For this review, take the finished solid that the model builds, in its own axes (mm). Face numbers are marked on the shaded views. Round coordinates to 2 decimals unless told otherwise and drop trailing zeros. Write each loop counter-clockwise with the first axis right and the second up, starting at its lowest first coordinate (ties: lowest second). Pieces come first, ordered by that corner, then holes. Notation, with made-up numbers: M 45,-28.75 L 58,-28.75 A16 cw 58,-7.75 Z; hole C 39.25,-38.5 d4. An arc over 180 degrees is marked long. Answer in a Markdown table with one row per item.
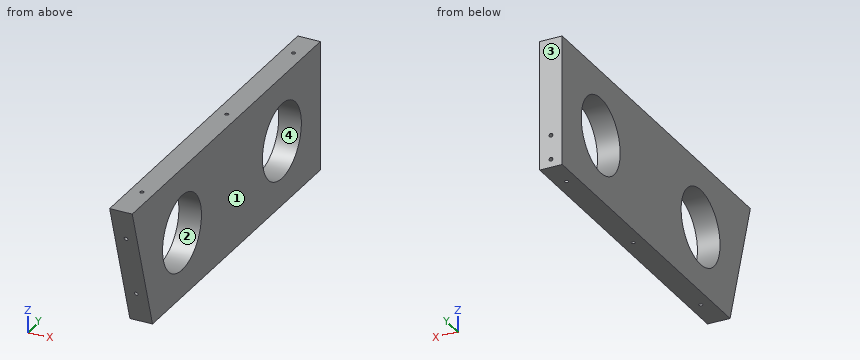
```python
from build123d import *

# Parameters (mm, degrees)
SKETCH1_W           = 19.05
SKETCH1_H           = 270.042121692
BOSS_EXTRUDE1_DEPTH = 33.95
SKETCH2_W           = 19.05
SKETCH2_H           = 270.042121692
BOSS_EXTRUDE2_DEPTH = 75.35
BOSS_EXTRUDE3_DEPTH = 19.05
HOLE1_D             = 3.175
HOLE1_DEPTH         = 31.75
HOLE1_CSINK_D       = 10.16
HOLE1_CSINK_ANGLE   = 82
HOLE1_TIP           = 0.953866233
HOLE3_D             = 3.175
HOLE3_DEPTH         = 31.75
HOLE3_CSINK_D       = 10.16
HOLE3_CSINK_ANGLE   = 82
HOLE3_TIP           = 0.953866233
HOLE4_D             = 3.175
HOLE4_DEPTH         = 31.75
HOLE4_CSINK_D       = 10.16
HOLE4_CSINK_ANGLE   = 82
HOLE4_TIP           = 0.953866233
HOLE5_D             = 3.175
HOLE5_DEPTH         = 31.75
HOLE5_CSINK_D       = 10.16
HOLE5_CSINK_ANGLE   = 82
HOLE5_TIP           = 0.953866233
HOLE6_D             = 63.5
HOLE6_DEPTH         = 19.05


with BuildPart() as part:
    # Sketch1 → Boss-Extrude1 (new body)
    with BuildSketch(Plane.XY):
        with Locations((-124.004465969, -292.321060846)):
            Rectangle(SKETCH1_W, SKETCH1_H)
    extrude(amount=BOSS_EXTRUDE1_DEPTH)

    # Sketch2 → Boss-Extrude2 (add)
    with BuildSketch(Plane.XY.offset(33.95)):
        with Locations((-124.004465969, -292.321060846)):
            Rectangle(SKETCH2_W, SKETCH2_H)
    extrude(amount=BOSS_EXTRUDE2_DEPTH)

    # Sketch3 → Boss-Extrude3 (add, through all)
    with BuildSketch(Plane.ZY.offset(133.529465969)):
        Polygon((109.3, -427.342121692), (109.3, -464.26606302), (0, -431.185843453), (0, -427.342121692), align=None)
    extrude(amount=-BOSS_EXTRUDE3_DEPTH)

    # Hole1
    with Locations(Plane(origin=(-124.004465969, 10.424290059, 122), x_dir=(-1, 0, 0), z_dir=(0, 0, 1))):
        with Locations((113.649999994, 128.807623392), (113.649999994, 23.940956725), (-94.599999994, 161.374290059), (94.599999994, 161.374290059), (0, 161.374290059), (0, 193.124290059), (0, 440.553783621), (0, 301.970350905), (40.979166666, 301.970350905), (166.795833328, 301.970350905), (207.774999994, 440.553783621), (207.774999994, 333.02141023), (207.774999994, 225.48903684), (207.774999994, 137.424290059), (207.774999994, 10.424290059), (-207.774999994, 10.424290059), (-207.774999994, 137.424290059), (-207.774999994, 225.48903684), (-207.774999994, 333.02141023), (-207.774999994, 440.553783621), (-166.795833328, 301.970350905), (-40.979166666, 301.970350905), (-113.649999994, 23.940956725), (-113.649999994, 128.807623392)):
            CounterSinkHole(HOLE1_D / 2, HOLE1_CSINK_D / 2, depth=HOLE1_DEPTH, counter_sink_angle=HOLE1_CSINK_ANGLE)
            with Locations((0, 0, -(HOLE1_DEPTH + HOLE1_TIP / 2))):  # 118° drill point
                Cone(0, HOLE1_D / 2, HOLE1_TIP, mode=Mode.SUBTRACT)

    # Hole3
    with Locations(Plane(origin=(-124.004465969, -144.6, -155.286738577), x_dir=(-1, 0, 0), z_dir=(0, 1, 0))):
        with Locations((0, 162.086738577), (0, 182.486738577)):
            CounterSinkHole(HOLE3_D / 2, HOLE3_CSINK_D / 2, depth=HOLE3_DEPTH, counter_sink_angle=HOLE3_CSINK_ANGLE)
            with Locations((0, 0, -(HOLE3_DEPTH + HOLE3_TIP / 2))):  # 118° drill point
                Cone(0, HOLE3_D / 2, HOLE3_TIP, mode=Mode.SUBTRACT)

    # Hole4
    with Locations(Plane(origin=(-124.004465969, 10.424290059, -12.7), x_dir=(1, 0, 0), z_dir=(0, 0, -1))):
        with Locations((-207.774999994, 333.02141023), (-207.774999994, 225.48903684), (-207.774999994, 137.424290059), (-172.166666661, 4.074290059), (-146.083333327, 4.074290059), (-94.599999994, 161.374290059), (0, 161.374290059), (94.599999994, 161.374290059), (146.083333327, 4.074290059), (172.166666661, 4.074290059), (207.774999994, 137.424290059), (207.774999994, 225.48903684), (207.774999994, 333.02141023), (166.795833328, 301.970350905), (40.979166666, 301.970350905), (-40.979166666, 301.970350905), (-166.795833328, 301.970350905), (0, 193.124290059), (0, 301.970350905), (0, 412.366411751), (-126.349999994, 106.824290059), (-126.349999994, 58.624290059), (126.349999994, 58.624290059), (126.349999994, 106.824290059)):
            CounterSinkHole(HOLE4_D / 2, HOLE4_CSINK_D / 2, depth=HOLE4_DEPTH, counter_sink_angle=HOLE4_CSINK_ANGLE)
            with Locations((0, 0, -(HOLE4_DEPTH + HOLE4_TIP / 2))):  # 118° drill point
                Cone(0, HOLE4_D / 2, HOLE4_TIP, mode=Mode.SUBTRACT)

    # Hole5
    with Locations(Plane(origin=(-124.004465969, -363.229637966, -268.375064111), x_dir=(1, 0, 0), z_dir=(0, -0.957123977, -0.289678603))):
        with Locations((207.774999994, 613.051808534), (-207.774999994, 613.051808534), (-207.774999994, 456.277103296), (-207.774999994, 769.826513772), (-108.649999997, 456.277103296), (-108.649999997, 630.126513772), (-108.649999997, 769.826513772), (-207.774999994, 362.200879148), (-207.774999994, 305.10273792), (0, 305.10273792), (0, 362.200879148), (207.774999994, 305.10273792), (207.774999994, 362.200879148), (108.649999997, 769.826513772), (108.649999997, 630.126513772), (108.649999997, 456.277103296), (207.774999994, 769.826513772), (207.774999994, 456.277103296)):
            CounterSinkHole(HOLE5_D / 2, HOLE5_CSINK_D / 2, depth=HOLE5_DEPTH, counter_sink_angle=HOLE5_CSINK_ANGLE)
            with Locations((0, 0, -(HOLE5_DEPTH + HOLE5_TIP / 2))):  # 118° drill point
                Cone(0, HOLE5_D / 2, HOLE5_TIP, mode=Mode.SUBTRACT)

    # Hole6
    with Locations(Plane.ZY.offset(133.529465969)):
        with Locations((54.65, -220.048030423), (54.65, -383.056061933)):
            Hole(HOLE6_D / 2, depth=HOLE6_DEPTH)


solid = part.part
```
Q1. Take a section at D-D (z = 74.5). State the section outline as (x, y) points, then the cut area to 3 significant figures.
Found:
| item | result |
|---|---|
| outline | M -133.53,-453.73 L -114.48,-453.73 L -114.48,-407.84 L -133.53,-407.84 Z; M -133.53,-358.28 L -114.48,-358.28 L -114.48,-244.83 L -133.53,-244.83 Z; M -133.53,-195.27 L -114.48,-195.27 L -114.48,-157.3 L -133.53,-157.3 Z |
| area | 3,760 mm² |
Q2. Take a section at B-B (y = -370). State the section outline as (x, z) points.
Found:
| item | result |
|---|---|
| outline | M -133.53,0 L -114.48,0 L -114.48,25.71 L -133.53,25.71 Z; M -133.53,83.59 L -114.48,83.59 L -114.48,109.3 L -133.53,109.3 Z |
Q3. Take a section at A-A (z = 49.5). State the section outline as (x, y) points, then the cut area to 3 significant figures.
Found:
| item | result |
|---|---|
| outline | M -133.53,-446.17 L -114.48,-446.17 L -114.48,-414.39 L -133.53,-414.39 Z; M -133.53,-351.73 L -114.48,-351.73 L -114.48,-251.38 L -133.53,-251.38 Z; M -133.53,-188.72 L -114.48,-188.72 L -114.48,-157.3 L -133.53,-157.3 Z |
| area | 3,120 mm² |
Q4. Insertion check: P1, Ø3.5, axis at x = -124, y = -291.55, coming from the -Z side; P2, Ø2.5, axis at x = -124, y = -430.13, coming from the +Z side; P3, Ø1.9, axis at x = -124, z = 6.8, coming from the +Y side; P4, Ø1, axis at x = -131.5, z = 40.5, coming from the -Y side. Each pin has a flat end and moves straight along its axis. Give the tip position at first contact, or say it passes through.
Found:
| item | result |
|---|---|
| P1 | z = 0 |
| P2 | z = 90.05 |
| P3 | y = -176.73 |
| P4 | y = -443.59 |
Q5. Mouldability with a two-part tool opening along Y and no side actions: class the marked faces 1, 2, 3 and 4 as +Y half, -Y half, draft (parallel to the pull), parting line (faces both ways), or undercut.
Found:
| item | result |
|---|---|
| face 1 | draft |
| face 2 | undercut |
| face 3 | +Y half |
| face 4 | undercut |
Q6. Take a section at C-C (y = -246). State the section outline as (x, z) points, then the cut area to 3 significant figures.
Found:
| item | result |
|---|---|
| outline | M -133.53,0 L -114.48,0 L -114.48,36.36 L -133.53,36.36 Z; M -133.53,72.94 L -114.48,72.94 L -114.48,109.3 L -133.53,109.3 Z |
| area | 1,390 mm² |
Q7. For probe 1 along Y at (x, z) = (-119.25, 70); probe 2 along Y at (x, z) = (-123.5, 75.5); probe 3 along X at (y, z) = (-168, 27), list the stretches that pass through material, from the lowest coordinate up.
Found:
| item | result |
|---|---|
| probe 1 | -452.37 to -410.85, -355.26 to -247.84, -192.26 to -157.3 |
| probe 2 | -454.04 to -407, -359.11 to -243.99, -196.1 to -157.3 |
| probe 3 | -133.53 to -125.58, -122.43 to -114.48 |
